CAD build for the part. Positions are in the model's coordinates, mm. Face numbers are marked on the shaded views. A direction names the side the tool comes from. Coordinates: 2 decimals unless noted, no trailing zeros. Write each loop counter-clockwise with the first axis right and the second up, starting at its lowest first coordinate (ties: lowest second). Pieces come first, ordered by that corner, then holes.
Autodesk Inventor part; units mm, degrees
ref_plane "YZ Plane" through (0, 0, 0) normal (1, 0, 0) x (0, 1, 0)
ref_plane "XZ Plane" through (0, 0, 0) normal (0, 1, 0) x (-1, 0, 0)
ref_plane "XY Plane" through (0, 0, 0) normal (0, 0, 1) x (1, 0, 0)
sketch "Sketch1" plane through (0, 0, 0) normal (1, 0, 0) x (0, 1, 0)
  circle A0 centre (0, 0) radius 70
  line L0 (0, 0) -> (66.7602, 21.0494) construction
  line L1 (66.7602, -21.0494) -> (0, 0) construction
  line L2 (66.7602, -21.0494) -> (66.7602, 21.0494) construction
  circle A1 centre (66.7602, 21.0494) radius 1.65
  circle A2 centre (66.7602, -21.0494) radius 1.65
  circle A3 centre (0, 0) radius 57.5
  line L3 (64.3545, 28.6791) -> (-26.6041, 0)
  line L4 (-26.6041, 0) -> (64.3545, -28.6791)
  line L5 (74.7602, -21.0494) -> (74.7602, 21.0494)
  arc A4 (74.7602, 21.0494) -> (64.3545, 28.6791) centre (66.7602, 21.0494) ccw
  arc A5 (64.3545, -28.6791) -> (74.7602, -21.0494) centre (66.7602, -21.0494) ccw
  circle A6 centre (0, 0) radius 64.5
  point P0 (66.7602, 0)
  point P1 (51.8997, 24.7522)
  point P2 (51.8997, -24.7522)
  point P3 (58.6341, 26.8755)
  point P4 (58.6341, -26.8755)
  dimension "d0" = 140
  dimension "d1" = 35
  dimension "d2" = 3.3
  dimension "d3" = 3.3
  dimension "d4" = 115
  dimension "d5" = 8
  dimension "d6" = 8
  dimension "d7" = 7
extrude "Extrusion1" add sketch "Sketch1" against normal blind 7 contours A0 A2 L4 A6 L3 A1 | A0 A1 L3 A4 L5 A5 L4 A2 | A6 L4 A3 L3 picked at (61.9464, 3.0696)
extrude "Extrusion2" add sketch "Sketch1" along normal blind 30 contours A6 L4 A3 L3 picked at (61.9464, 3.0696)
fillet "Fillet1" radius 5 2 edges at (30, 55.2669, 25.8138) (30, 55.2669, -25.8138)
chamfer "Chamfer1" distance 2 angle 45 1 edges at (0, 64.5, 0)
sketch "Sketch2" plane through (0, 0, 0) normal (1, 0, 0) x (0, 0, -1)
  arc A0 (27.4814, 60.5559) -> (-27.4814, 60.5559) centre (0, 0) ccw
  line L0 (27.4814, 60.5559) -> (28.6791, 64.3545)
  arc A1 (28.6791, 64.3545) -> (21.0494, 74.7602) centre (21.0494, 66.7602) ccw
  line L1 (21.0494, 74.7602) -> (-21.0494, 74.7602)
  arc A2 (-21.0494, 74.7602) -> (-28.6791, 64.3545) centre (-21.0494, 66.7602) ccw
  line L2 (-28.6791, 64.3545) -> (-27.4814, 60.5559)
  circle A3 centre (-21.0494, 66.7602) radius 1.65
  circle A4 centre (21.0494, 66.7602) radius 1.65
  circle A5 centre (-21.0494, 66.7602) radius 2.9
  circle A6 centre (21.0494, 66.7602) radius 2.9
  dimension "d16" = 5.8
  dimension "d17" = 5.8
extrude "Extrusion3" cut sketch "Sketch2" against normal blind 4 contours A3 | A4 | A5 | A6
sketch "Sketch3" plane through (-7, 0, 0) normal (-1, 0, 0) x (0, 0, 1)
  arc A0 (24.7522, 51.8997) -> (-24.7522, 51.8997) centre (0, 0) ccw
  line L0 (24.7522, 51.8997) -> (28.6791, 64.3545)
  arc A1 (28.6791, 64.3545) -> (21.0494, 74.7602) centre (21.0494, 66.7602) ccw
  line L1 (21.0494, 74.7602) -> (-21.0494, 74.7602)
  arc A2 (-21.0494, 74.7602) -> (-28.6791, 64.3545) centre (-21.0494, 66.7602) ccw
  line L2 (-28.6791, 64.3545) -> (-24.7522, 51.8997)
  circle A3 centre (21.0494, 66.7602) radius 1.65
  circle A4 centre (-21.0494, 66.7602) radius 1.65
  arc A5 (25.4764, 50.206) -> (-25.4764, 50.206) centre (0, 0) ccw
  line L3 (25.4764, 50.206) -> (29.8236, 63.9937)
  arc A6 (29.8236, 63.9937) -> (21.0494, 75.9602) centre (21.0494, 66.7602) ccw
  line L4 (21.0494, 75.9602) -> (-21.0494, 75.9602)
  arc A7 (-21.0494, 75.9602) -> (-29.8236, 63.9937) centre (-21.0494, 66.7602) ccw
  line L5 (-29.8236, 63.9937) -> (-25.4764, 50.206)
  line L6 (0, -26.6041) -> (-28.6791, 64.3545)
  line L7 (28.6791, 64.3545) -> (0, -26.6041)
  point P0 (24.3877, 50.7438)
  point P1 (-24.3877, 50.7438)
  dimension "d20" = 1.2
extrude "Extrusion4" add sketch "Sketch3" against normal blind 20 contours L7 A5 L6 A0
sketch "Sketch4" plane through (30, 0, 0) normal (1, 0, 0) x (0, 0, -1)
  line L0 (22.2357, 60.5461) -> (20.1282, 53.8619)
  arc A0 (22.2357, 60.5461) -> (-22.2357, 60.5461) centre (0, 0) ccw
  line L1 (-20.1282, 53.8619) -> (-22.2357, 60.5461)
  line L2 (-20.1282, 53.8619) -> (-22.2357, 60.5461)
  spline S0 degree 3 poles (-22.2357, 60.5461) (-22.8268, 60.329) (-23.4536, 60.088) (-24.6005, 59.6276) (-25.1209, 59.4087) (-25.9393, 59.0559) (-26.2925, 58.8984) (-26.7214, 58.7049) (-26.8341, 58.6531) (-26.8662, 58.6384) (-26.8693, 58.6369) (-26.8724, 58.6355) (-26.8755, 58.6341) knots 0.753525 0.753525 0.753525 0.753525 0.94243 0.94243 1.131336 1.131336 1.319777 1.319777 1.476719 1.476719 1.476719 1.491826 1.491826 1.491826 1.491826
  line L3 (-26.8755, 58.6341) -> (-24.7522, 51.8997)
  line L4 (22.2357, 60.5461) -> (20.1282, 53.8619)
  spline S1 degree 8 poles (20.1282, 53.8619) (20.3348, 53.7847) (20.5411, 53.7066) (20.7457, 53.6281) (20.9475, 53.5496) (21.1456, 53.4716) (21.339, 53.3945) (21.5271, 53.3186) (21.9974, 53.1268) (22.2707, 53.0133) (22.5278, 52.9047) (22.768, 52.8016) (22.9911, 52.7046) (23.1973, 52.6138) (23.3871, 52.5293) (23.8704, 52.3122) (24.1287, 52.1937) (24.34, 52.0952) (24.5063, 52.0167) (24.6296, 51.9582) (24.7112, 51.9192) (24.7522, 51.8997) (24.7522, 51.8997) knots 0 0 0 0 0 0 0 0 0 0.185394 0.185394 0.185394 0.185394 0.185394 0.185394 0.185394 0.478501 0.478501 0.478501 0.478501 0.478501 0.478501 0.478501 1 1 1 1 1 1 1 1 1
  line L5 (24.7522, 51.8997) -> (26.8755, 58.6341)
  arc A1 (24.3877, 50.7438) -> (-24.3877, 50.7438) centre (0, 0) ccw
  arc A2 (25.6872, 53.4477) -> (-25.6872, 53.4477) centre (0, 0) ccw
  line L6 (-24.7522, 51.8997) -> (-24.3877, 50.7438)
  line L7 (24.7522, 51.8997) -> (24.3877, 50.7438)
  point P0 (20.6702, 55.5809)
  point P1 (-25.2986, 53.6328)
  point P2 (25.2986, 53.6328)
  dimension "d23" = 3
extrude "Extrusion5" cut sketch "Sketch4" against normal through all contours A2 L5 S1 L0 | L0 S1 L7 A1 L6 L3 A2
properties part number "SEGURO_CANALETA" material "Steel, Mild, Welded"
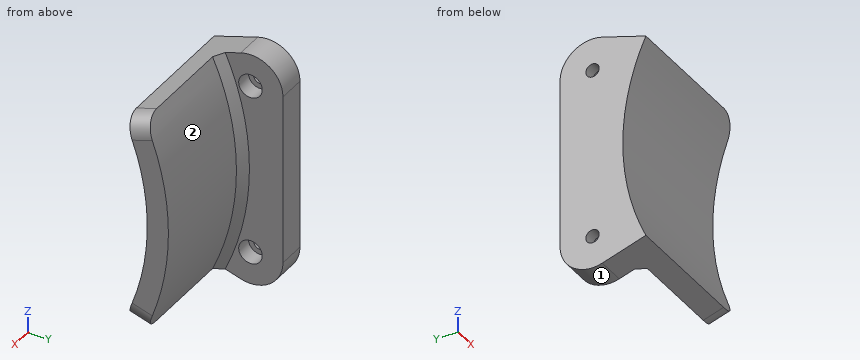
Item 1: Saw through at A-A, the plane y = 69. Write the cut outline in (x, z).
Item 2: Flat gauge pins, fed straight in: pin 1 Ø4.5 at (y, z) = (69, 1) entering from +X; pin 2 Ø3 at (x, y) = (15, 59) entering from -Z; pin 3 Ø6 at (x, z) = (4.5, -22) entering from -Y. Where does each tip first touch, or does it go through?
Item 3: Saw through at B-B, the plane x = 11. Write the cut outline in (y, z), and give its area (3 significant figures).
Item 4: Which spindle directions (+Z, -Z, +X, -X, +Y, -Y) get a long thin tool onto all of the face, cutting with end or side? Do the marked faces 1 and 2. Say none if no direction does.
Item 5: Wall check: line 1 along X through (y, z) = (66.25, 23); line 2 along Y through (x, z) = (6, -18.5); line 3 along X through (y, z) = (70, 13). Give the ranges that are in metal, low to high.
Working result:
1. outline: (-7, -28.73) - (0, -28.73) - (0, -22.89) - (-4, -22.89) - (-4, -19.21) - (0, -19.21) - (0, 19.21) - (-4, 19.21) - (-4, 22.89) - (0, 22.89) - (0, 28.73) - (-7, 28.73) - close
2. pin 1: stops at x = 0
2. pin 2: stops at z = -26.88
2. pin 3: stops at y = 53.77
3. outline: (53.63, -25.3) - (58.63, -26.88) arc R64.5 ccw to (58.63, 26.88) - (53.63, 25.3) arc R59.3 cw to start
3. area: 280 mm2
4. face 1: -Z, +X, -X
4. face 2: +X, +Y
5. line 1: x = -7 to -4
5. line 2: y = 56.34 to 61.79
5. line 3: x = -7 to 0
